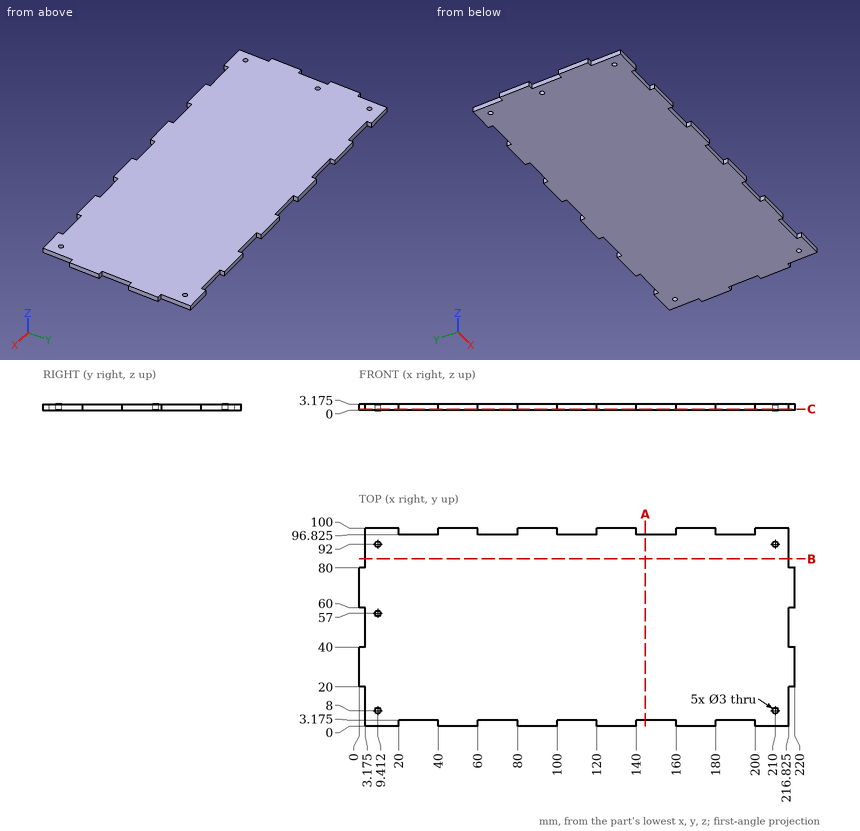
Can you work these out from the drawing? Everything is in mm from the part's minimum corner. Round coordinates to 2 decimals unless told otherwise and drop trailing zeros. Loops run counter-clockwise (first coordinate to the right, second up) from the corner with the lowest first, then second, coordinate; pieces in that order, holes last. Notation, with made-up numbers: (-16.75, -2) -> (-9.75, -2) arc R30 ccw to (-9.75, 35) -> close; hole circle Ø9 at (-34.75, 41). An arc over 180 degrees is marked (long way). Put each result on its own line as item: value.
Q1. Please list where these lines run through material, in increasing order: line 1 (Y direction, x = 210, z = 1.6); line 2 (Y direction, x = 9.5, z = 0.35); line 3 (Y direction, x = 70, z = 0.95) (1 decimal). Write a range as from..to.
Checks:
line 1: 0..6.5, 9.5..90.5, 93.5..100
line 2: 0..6.5, 9.5..55.5, 58.5..90.5, 93.5..100
line 3: 3.2..96.8
Q2. I want a section at B-B on y = 84.5. Write out the boundary of the cut face in (x, z) (1 decimal).
Checks:
outline: (3.2, 0) -> (216.8, 0) -> (216.8, 3.2) -> (3.2, 3.2) -> close
Q3. I want a section at A-A on x = 144.5. Write out the boundary of the cut face in (y, z) (1 decimal).
Checks:
outline: (3.2, 0) -> (96.8, 0) -> (96.8, 3.2) -> (3.2, 3.2) -> close
Q4. I want a section at C-C on z = 0.55. Give the number of separate pieces and of enclosed holes in the cut face, and give its area (3 significant figures).
Checks:
separate pieces: 1
enclosed holes: 5
area: 20,900 mm2
Q5. For pin 1 Ø1.6 at (x, z) = (219, 1.5) entering from -Y; pin 2 Ø1 at (y, z) = (88, 2) entering from +X (3 decimals), each with a flat end and sliding along its axis, tell me the tip position at first contact or that it passes through.
Checks:
pin 1: y = 20
pin 2: x = 216.825
